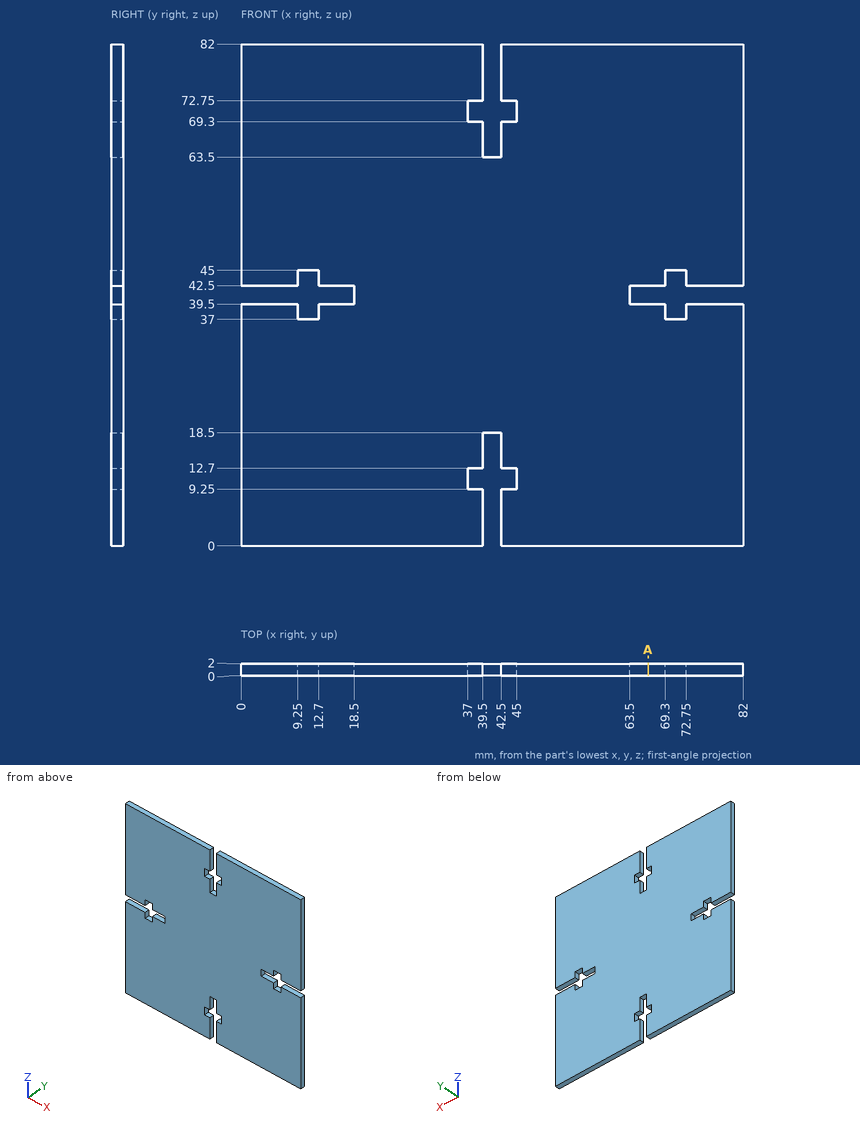
Drawing for the job (mm, zero at the part's lowest x, y, z). Round coordinates to 2 decimals unless told otherwise and drop trailing zeros. Order: outer loops, then holes, each group sorted by start corner. A loop starts at its lowest first (then second) coordinate and runs counter-clockwise, first axis right, second up.
Item 1: Probe line 1 along Z through (x, y) = (44, 0.55); line 2 along X through (y, z) = (1.35, 76). List the from-to ranges inside material, lowest first.
Item 2: Saw through at A-A on x = 66.5. Write the cut outline in (y, z).
Item 3: Pin check, flat tip, straight feed: pin 1 (1 mm diameter, centred on x = 40.5, y = 1, fed in from -Z). Stop position of the tip, or through.
Reported:
1. line 1: z = 0 to 9.25, 12.7 to 69.3, 72.75 to 82
1. line 2: x = 0 to 39.5, 42.5 to 82
2. outline: (0, 0) - (2, 0) - (2, 39.5) - (0, 39.5) - close; (0, 42.5) - (2, 42.5) - (2, 82) - (0, 82) - close
3. pin 1: stops at z = 18.5
